```python
from build123d import *

# Parameters (mm, degrees)
F1_DEPTH = 88.9
F2_R     = 12.7
F2_W     = 85.725
F2_H     = 41.275
F2_R_2   = 4.7625
F3_DEPTH = 62.862793


with BuildPart() as f1:
    # F0 (on Right) → F1 (new body, symmetric)
    with BuildSketch(Plane.YZ):
        Polygon((88.9, 88.9), (0, 0), (8.980256, 0), (88.9, 79.919744), align=None)
    extrude(amount=F1_DEPTH, both=True)

    # F2 (on face) → F3 (cut, through all)
    with BuildSketch(Plane(origin=(0, 0, 0), x_dir=(1, 0, 0), z_dir=(0, -0.707107, 0.707107))):
        with Locations((50.8, 87.623586)):
            Circle(F2_R)
        with Locations((-50.8, 87.623586)):
            Circle(F2_R)
        with Locations((0, 41.275)):
            Rectangle(F2_W, F2_H)
        with Locations((0, 87.623586)):
            Circle(F2_R_2)
    extrude(amount=-F3_DEPTH, mode=Mode.SUBTRACT)


solid = f1.part
```
Can you work these out from the model? Positions are in its coordinate system, mm. A direction names the side the tool comes from. Give positions to 0.01 mm unless a question says otherwise; leave off trailing zeros. Write each loop counter-clockwise with the first axis right and the second up, starting at its lowest first coordinate (ties: lowest second). Pieces come first, ordered by that corner, then holes. Notation, with made-up numbers: (0, 70) - (19, 70) arc R28 ccw to (19, 106) - close; hole circle Ø9 at (50.5, 20). An arc over 180 degrees is marked (long way). Write item = value, one per line. Start each with the question number.
1. Imagine slicing it at B-B (x = -2). Please give me the cut outline in (y, z).
2. Thinking about a two-plate mould opening in X: for faces 4 (the face through (-42.862, 31, 27)), 5 (the face through (88.9, 48, 41)), 6 (the face through (1, 88.9, 84)), which applies, released by +X, released by -X, zero draft, split by the parting line, or undercut?
3. Please list where these lines run through material, in increasing order: line 1 (X direction, y = 55.5, z = 52); line 2 (Z direction, x = 73.5, y = 70); line 3 (Z direction, x = 32.5, y = 77).
4. Imagine slicing it at D-D (y = 46.5). Please give me the cut outline in (x, z), and give its area (3 significant figures).
5. Imagine slicing it at C-C (z = 32). Please give me the cut outline in (x, y), and give its area (3 significant figures).
6. On a 3-axis mill with a long thin cutter (end or side, diameter ignored), from which of +Z, -Z, +X, -X, +Y, -Y can I reach the whole of each face in a straight line? I mean faces 1 (the face through (-0.6, 45.99, 41.57)), 2 (the face through (-0.6, 16.807, 12.379)), 3 (the face through (4.543, 65.184, 60.757)). Say none if no direction works.
7. Imagine slicing it at A-A (x = 20). Please give me the cut outline in (y, z).
8. For pin 1 (4 mm diameter, centred on x = 63.5, y = 49.5, fed in from -Z); pin 2 (5 mm diameter, centred on x = 58, y = 18, fed in from -Z); pin 3 (6 mm diameter, centred on x = 15.5, y = 13.5, fed in from +Z), each with a flat end and sliding along its axis, tell me the tip position at first contact or that it passes through.
Worked answers:
q1.outline = (0, 0) - (8.98, 0) - (19.08, 10.1) - (14.59, 14.59) - close; (43.78, 43.78) - (48.27, 39.29) - (63.39, 54.41) - (58.9, 58.9) - close; (65.02, 65.02) - (69.51, 60.53) - (88.9, 79.92) - (88.9, 88.9) - close
q2.face_4 = undercut
q2.face_5 = released by +X
q2.face_6 = zero draft
q3.line_1 = -88.9 to -55.95, -45.65 to 45.65, 55.95 to 88.9
q3.line_2 = 61.02 to 70
q3.line_3 = 68.02 to 77
q4.outline = (-88.9, 37.52) - (-42.86, 37.52) - (-42.86, 41.06) - (42.86, 41.06) - (42.86, 37.52) - (88.9, 37.52) - (88.9, 46.5) - (-88.9, 46.5) - close
q4.area = 1,290 mm2
q5.outline = (-88.9, 32) - (-42.86, 32) - (-42.86, 40.98) - (-88.9, 40.98) - close; (42.86, 32) - (88.9, 32) - (88.9, 40.98) - (42.86, 40.98) - close
q5.area = 827 mm2
q6.face_1 = -Z, -Y
q6.face_2 = +Z, +Y
q6.face_3 = none
q7.outline = (0, 0) - (8.98, 0) - (19.08, 10.1) - (14.59, 14.59) - close; (43.78, 43.78) - (48.27, 39.29) - (88.9, 79.92) - (88.9, 88.9) - close
q8.pin_1 = 38.52
q8.pin_2 = 6.52
q8.pin_3 = 14.59
